from build123d import *

# Parameters (mm, degrees)
BOSS_EXTRUDE1_START = 3.96875
SKETCH3_R           = 10.31875
BOSS_EXTRUDE1_DEPTH = 3.96875


with BuildPart() as part:
    # Sketch1 → Revolve1 (revolve)
    with BuildSketch(Plane.XY, mode=Mode.PRIVATE) as revolve1_sk:
        Polygon((-17.065625, -10.31875), (-1.984375, -10.31875), (-1.984375, -6.388443876), (-17.065625, -6.858), align=None)
    revolve(revolve1_sk.sketch.rotate(Axis((-17.065625, 0, 0), (1, 0, 0)), 270), axis=Axis((-17.065625, 0, 0), (1, 0, 0)))


with BuildPart() as body_2:
    # Mirror2: mirrored copy
    add(part.part.mirror(Plane(origin=(0, 0, 0), x_dir=(0, 0, 1), z_dir=(1, 0, 0))))


with BuildPart() as part_1:
    add(part.part)

    add(body_2.part)  # Boss-Extrude1 merges body 2
    # Sketch3 → Boss-Extrude1 (add)
    with BuildSketch(Plane(origin=(-1.984375, 0, 0), x_dir=(0, 0, -1), z_dir=(1, 0, 0)).offset(BOSS_EXTRUDE1_START)):
        with Locations(Location((0, 0, 0), (0, 0, 180))):
            Circle(SKETCH3_R)
    extrude(amount=-BOSS_EXTRUDE1_DEPTH)

    # Sketch8 → Cut-Revolve1 (revolve, cut)
    with BuildSketch(Plane.XY):
        Polygon((-17.065625, 0), (17.065625, 0), (17.065625, -6.858), (1.984375, -6.388443876), (1.984375, -3.365843876), (-1.984375, -3.365843876), (-1.984375, -6.388443876), (-17.065625, -6.858), align=None)
    revolve(axis=Axis((-17.065625, 0, 0), (1, 0, 0)), mode=Mode.SUBTRACT)


solid = part_1.part
Input: part model. Units: mm. Frame: model coordinates. Give positions to 0.01 mm unless a question says otherwise; leave off trailing zeros. Write each loop counter-clockwise with the first axis right and the second up, starting at its lowest first coordinate (ties: lowest second). Pieces come first, ordered by that corner, then holes.
Q1. Material intervals for probe 1 along Y at (x, z) = (0.85, 0); probe 2 along Z at (x, y) = (-14, -3.25); probe 3 along Y at (x, z) = (-10, -2.5), sorted ascending.
Q2. Section B-B, the plane z = -8.5. Output: boundary loops of the cut face in (x, y), plus the area to 3 significant figures.
Q3. Section D-D, the plane z = 8. Output: boundary loops of the cut face in (x, y), plus the area to 3 significant figures.
Q4. Section A-A, the plane x = -5. Output: boundary loops of the cut face in (y, z).
Q5. Section C-C, the plane x = -14.5. Output: boundary loops of the cut face in (y, z), plus the area to 3 significant figures.
Q6. First-contact query: P1, Ø1.5, axis at x = -7, y = -6, coming from the -Z side; P2, Ø3, axis at x = -9.5, y = -3, coming from the -Z side; P3, Ø6, axis at y = 0, z = 0, coming from the -X side; P4, Ø3, axis at y = 0.5, z = 4.5, coming from the +X side. Flat tips, straight axial feed; report the tip coordinate or a pass-through.
Q7. Pull-direction query (Z, two-part tool) for faces 1 (the face through (-17.066, 7, -2)), 2 (the face through (-1.984, 3, 3)), 3 (the face through (1.984, 3, 3)); classes: pulls with the +Z half, pulls with the -Z half, needs draft (parallel to the pull), parting line crosses it, or undercut.
Filled in:
1. probe 1: y = -10.32 to -3.37, 3.37 to 10.32
1. probe 2: z = -9.79 to -5.93, 5.93 to 9.79
1. probe 3: y = -10.01 to -6.15, 6.15 to 10.01
2. outline: (-17.07, -5.85) - (17.07, -5.85) - (17.07, 5.85) - (-17.07, 5.85) - close
2. area: 399 mm2
3. outline: (-17.07, -6.52) - (17.07, -6.52) - (17.07, 6.52) - (-17.07, 6.52) - close
3. area: 445 mm2
4. outline: circle Ø20.64 at (0, 0); hole circle Ø12.96 at (0, 0)
5. outline: circle Ø20.64 at (0, 0); hole circle Ø13.56 at (0, 0)
5. area: 190 mm2
6. P1: stops at z = -8.88
6. P2: stops at z = -10.21
6. P3: passes through
6. P4: stops at x = 1.98
7. face 1: needs draft
7. face 2: undercut
7. face 3: undercut
